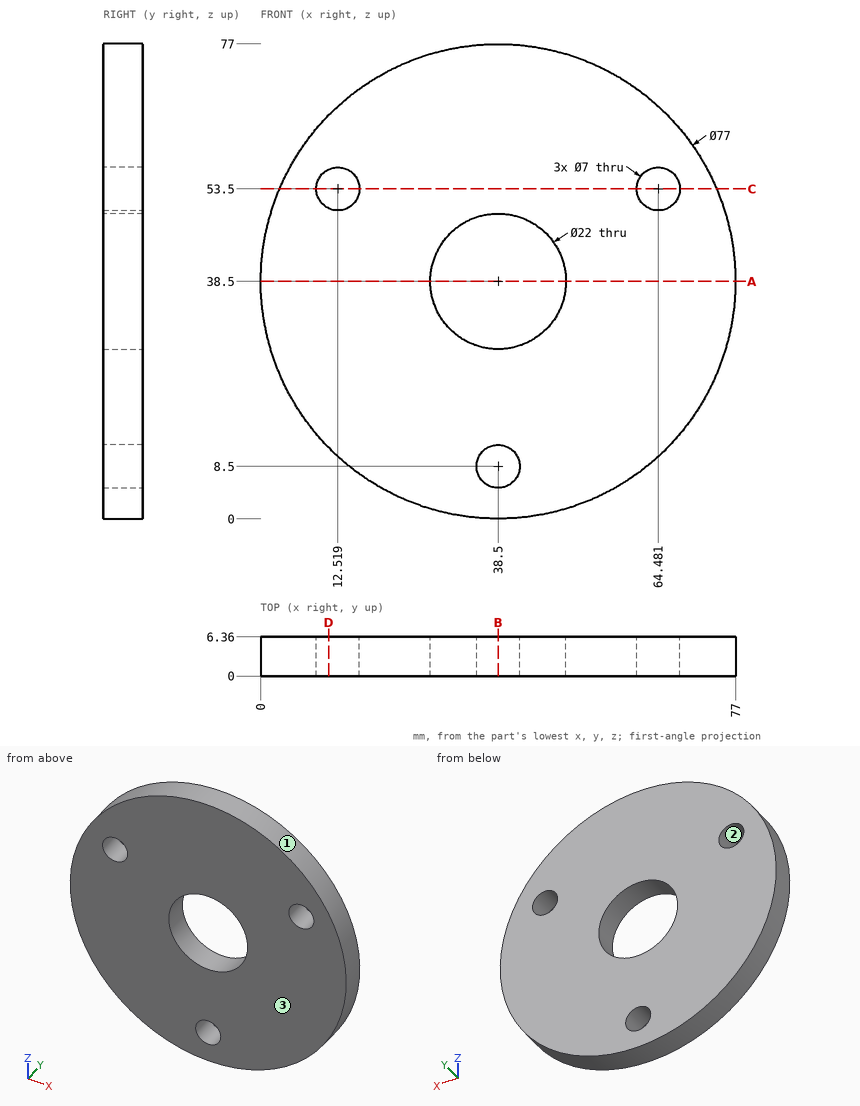
Study the drawing (mm; zero at the part's minimum x, y, z) and answer. Coordinates: 2 decimals unless noted, no trailing zeros. Loops run counter-clockwise (first coordinate to the right, second up) from the corner with the lowest first, then second, coordinate; pieces in that order, holes last. Notation, with made-up numbers: (48, -32) -> (86, -32) arc R27 ccw to (86, 7) -> close; hole circle Ø5 at (-3.75, 82). An arc over 180 degrees is marked (long way). Answer as CSV lines item,"result".
1) For a pull along X with two mould halves and no side action, classify the marked faces 1, 2 and 3 as released by +X, released by -X, zero draft, split by the parting line, or undercut.
A:
face 1,"split by the parting line"
face 2,"undercut"
face 3,"zero draft"
2) The part is cut by section B-B (x = 38.5). Give the vertices of the cut face in (y, z).
A:
outline,"(0, 0) -> (6.36, 0) -> (6.36, 5) -> (0, 5) -> close; (0, 12) -> (6.36, 12) -> (6.36, 27.5) -> (0, 27.5) -> close; (0, 49.5) -> (6.36, 49.5) -> (6.36, 77) -> (0, 77) -> close"
3) Flat-ended cylindrical pins translate along their axes: pin 1 (3 mm diameter, centred on y = 1.5, z = 15.5, fed in from -X); pin 2 (8 mm diameter, centred on x = 12.52, z = 53.5, fed in from +Y); pin 3 (1.5 mm diameter, centred on y = 5.5, z = 13, fed in from -X). Find the tip coordinate at first contact, or state that the pin passes through.
A:
pin 1,"stops at x = 6.56"
pin 2,"stops at y = 6.36"
pin 3,"stops at x = 9.01"
4) Straight lines are drawn through the part: probe 1 along Z at (x, y) = (38.5, 4.75); probe 2 along X at (y, z) = (4.5, 53.5); probe 3 along Z at (x, y) = (37, 5.25). For each, find the intervals that lie inside material, in ascending order.
A:
probe 1,"z = 0 to 5, 12 to 27.5, 49.5 to 77"
probe 2,"x = 3.04 to 9.02, 16.02 to 60.98, 67.98 to 73.96"
probe 3,"z = 0.03 to 5.34, 11.66 to 27.6, 49.4 to 76.97"
5) The part is cut by section D-D (x = 11). Give the vertices of the cut face in (y, z), and give its area (3 significant figures).
A:
outline,"(0, 11.56) -> (6.36, 11.56) -> (6.36, 50.35) -> (0, 50.35) -> close; (0, 56.65) -> (6.36, 56.65) -> (6.36, 65.44) -> (0, 65.44) -> close"
area,"303 mm²"
6) The part is cut by section A-A (z = 38.5). Give the vertices of the cut face in (x, y).
A:
outline,"(0, 0) -> (27.5, 0) -> (27.5, 6.36) -> (0, 6.36) -> close; (49.5, 0) -> (77, 0) -> (77, 6.36) -> (49.5, 6.36) -> close"
7) The part is cut by section C-C (z = 53.5). Give the vertices of the cut face in (x, y).
A:
outline,"(3.04, 0) -> (9.02, 0) -> (9.02, 6.36) -> (3.04, 6.36) -> close; (16.02, 0) -> (60.98, 0) -> (60.98, 6.36) -> (16.02, 6.36) -> close; (67.98, 0) -> (73.96, 0) -> (73.96, 6.36) -> (67.98, 6.36) -> close"
